Work out the finished part from the listing and answer in its coordinate system (mm). A direction names the side the tool comes from. Round coordinates to 2 decimals unless told otherwise and drop trailing zeros. Write each loop counter-clockwise with the first axis right and the second up, starting at its lowest first coordinate (ties: lowest second). Pieces come first, ordered by that corner, then holes.
1. A tool of negligible diameter and unlimited length cuts with its end or side. For faces 1 (the face through (-7, -27, 0)), 2 (the face through (3.724, 27.535, 3.697)), 3 (the face through (20, 0, 10)), 4 (the face through (21, -14, 15)), from which of +Z, -Z, +X, -X, +Y, -Y can it reach the whole face along a straight path? Write none if from no direction.
2. Find section A-A (y = -21). Write down the section's boundary in (x, z).
3. Straight lines are drawn through the part: probe 1 along Z at (x, y) = (-15, 28.15); probe 2 along Y at (x, z) = (-21, 17.75); probe 3 along Z at (x, y) = (-8, -26). For each, find the intervals that lie inside material, in ascending order.
4. Determine the mould class of faces 5 (the face through (-20.08, 27.54, 7.89)), 6 (the face through (-7, -27, 20)), 7 (the face through (43.5, -40, 12.6)) for opening direction X: pulls with the +X half, pulls with the -X half, needs draft (parallel to the pull), parting line crosses it, or undercut.
5. Flat-ended cylindrical pins translate along their axes: pin 1 Ø6 at (x, y) = (44, -2.5) entering from +Z; pin 2 Ø4 at (x, y) = (42, -36) entering from +Z; pin 3 Ø13 at (x, y) = (18.5, -38.5) entering from +Z. Find the tip coordinate at first contact, or state that the pin passes through.
6. Find section B-B (y = -83.5). Write down the section's boundary in (x, z), and give its area (3 significant figures).
```python
from build123d import *

# Parameters (mm, degrees)
BOSS_EXTRUDE2_DEPTH = 20
FILLET1_RADIUS      = 10
FILLET1_LENGTH      = 5
FILLET2_RADIUS      = 10
FILLET2_LENGTH      = 5
SKETCH5_R           = 1
SKETCH5_R_2         = 5.5
CUT_EXTRUDE5_DEPTH  = 69.007352544
CUT_EXTRUDE7_DEPTH  = 25
FILLET5_R           = 10
BOSS_EXTRUDE5_DEPTH = 60
SKETCH13_R          = 2.1
CUT_EXTRUDE8_DEPTH  = 60
BOSS_EXTRUDE6_START = 78
BOSS_EXTRUDE6_DEPTH = 78


with BuildPart() as part:
    # Sketch1 → Boss-Extrude2 (new body)
    with BuildSketch(Plane.XY):
        Polygon((-25, 30), (25, 30), (25, -30), (-25, -30), (-25, -25), (-20, -25), (20, -25), (20, 25), (-20, 25), (-25, 25), align=None)
    extrude(amount=BOSS_EXTRUDE2_DEPTH)

    # Fillet1: full round fillet: the end face becomes a half cylinder, R = half its width
    fillet1_face = Plane((-25, 27.5, 10), x_dir=(0, -1, 0), z_dir=(-1, 0, 0))  # on the end face: x along it, z out of the body
    fillet1_slab = fillet1_face.offset(-FILLET1_RADIUS / 2) * Box(FILLET1_LENGTH, 2 * FILLET1_RADIUS, FILLET1_RADIUS, mode=Mode.PRIVATE)  # the body's end, R deep
    fillet1_round = Plane((-15, 27.5, 10), x_dir=(-1, 0, 0), z_dir=(0, -1, 0)) * Cylinder(FILLET1_RADIUS, FILLET1_LENGTH, mode=Mode.PRIVATE)  # its axis R under the face
    add(fillet1_slab - fillet1_round, mode=Mode.SUBTRACT)

    # Fillet2: full round fillet: the end face becomes a half cylinder, R = half its width
    fillet2_face = Plane((-25, -27.5, 10), x_dir=(0, -1, 0), z_dir=(-1, 0, 0))  # on the end face: x along it, z out of the body
    fillet2_slab = fillet2_face.offset(-FILLET2_RADIUS / 2) * Box(FILLET2_LENGTH, 2 * FILLET2_RADIUS, FILLET2_RADIUS, mode=Mode.PRIVATE)  # the body's end, R deep
    fillet2_round = Plane((-15, -27.5, 10), x_dir=(-1, 0, 0), z_dir=(0, -1, 0)) * Cylinder(FILLET2_RADIUS, FILLET2_LENGTH, mode=Mode.PRIVATE)  # its axis R under the face
    add(fillet2_slab - fillet2_round, mode=Mode.SUBTRACT)

    # Sketch5 → Cut-Extrude5 (cut, through all)
    with BuildSketch(Plane(origin=(0, 30, 0), x_dir=(1, 0, 0), z_dir=(0, 1, 0))):
        with Locations(Location((-15, -3, 0), (0, 0, 180))):
            Circle(SKETCH5_R)
        with Locations(Location((-22, -10, 0), (0, 0, 180))):
            Circle(SKETCH5_R)
        with Locations(Location((-15, -17, 0), (0, 0, 180))):
            Circle(SKETCH5_R)
        with Locations(Location((-8, -10, 0), (0, 0, 180))):
            Circle(SKETCH5_R)
        with Locations(Location((-15, -10, 0), (0, 0, 180))):
            Circle(SKETCH5_R_2)
    extrude(amount=-CUT_EXTRUDE5_DEPTH, mode=Mode.SUBTRACT)

    # Sketch10 → Cut-Extrude7 (cut)
    with BuildSketch(Plane(origin=(25, 0, 0), x_dir=(0, 0, -1), z_dir=(1, 0, 0))):
        Polygon((-15, 28.180148829), (-15, -28.180148829), (-15, -30), (-20, -30), (-20, 30), (-15, 30), align=None)
        Polygon((-5, 28.180148829), (-5, -28.180148829), (-5, -30), (0, -30), (0, 30), (-5, 30), align=None)
    extrude(amount=-CUT_EXTRUDE7_DEPTH, mode=Mode.SUBTRACT)

    # Fillet5
    # the kernel refuses this fillet: 10 mm, written as the material it adds along each edge
    with BuildSketch(Plane(origin=(0, 25, 15), x_dir=(1, 0, 0), z_dir=(0, 1, 0)), Plane(origin=(0, -30, 15), x_dir=(1, 0, 0), z_dir=(0, 1, 0)), Plane(origin=(0, -25, 5), x_dir=(1, 0, 0), z_dir=(0, -1, 0))) as fillet5_piece_1:
        with BuildLine():
            CenterArc((8.660254038, -10), FILLET5_R, 90, 60)
            Line((0, -5), (-0.173205081, -4.9))
            ThreePointArc((-0.173205081, -4.9), (-0.2, -2.5), (-0.2, 0))
            Line((-0.2, 0), (0, 0.2))
            Line((0, 0.2), (8.660254038, 0.2))
            Line((8.660254038, 0.2), (8.660254038, 0))
        make_face()
    extrude(amount=5)
    with BuildSketch(Plane(origin=(0, 30, 5), x_dir=(0, 0, -1), z_dir=(0, -1, 0))) as fillet5_piece_2:
        with BuildLine():
            CenterArc((10, 8.660254038), FILLET5_R, 180, 60)
            Line((0, 8.660254038), (-0.2, 8.660254038))
            Line((-0.2, 8.660254038), (-0.2, 0))
            Line((-0.2, 0), (0, -0.2))
            ThreePointArc((0, -0.2), (2.5, -0.2), (4.9, -0.173205081))
            Line((4.9, -0.173205081), (5, 0))
        make_face()
    extrude(amount=5)

    # Sketch12 → Boss-Extrude5 (add)
    with BuildSketch(Plane.XZ.offset(30)):
        with BuildLine():
            Line((56.226298398, -3.359735054), (61.222506141, 5.302707337))
            ThreePointArc((61.222506141, 5.302707337), (43.74904955, 12.533728595), (25, 15))
            Line((25, 15), (25, 5))
            ThreePointArc((25, 5), (41.16297375, 2.873903962), (56.226298398, -3.359735054))
        make_face()
    extrude(amount=-BOSS_EXTRUDE5_DEPTH)

    # Sketch13 → Cut-Extrude8 (cut)
    with BuildSketch(Plane(origin=(2.920998947, 0, 10.910870277), x_dir=(-0.9659824633840055, 0, 0.2586075800021504), z_dir=(-0.2586075800021504, 0, -0.9659824633840055))):
        with Locations((-39.019497435, 15)):
            Circle(SKETCH13_R)
        with Locations((-39.019497435, 0)):
            Circle(SKETCH13_R)
        with Locations((-39.019497435, -15)):
            Circle(SKETCH13_R)
    extrude(amount=-CUT_EXTRUDE8_DEPTH, mode=Mode.SUBTRACT)

    # Sketch14 → Boss-Extrude6 (add)
    with BuildSketch(Plane.XZ.offset(30).offset(BOSS_EXTRUDE6_START)):
        with BuildLine():
            Line((61.222506141, 5.302707337), (56.226298398, -3.359735054))
            ThreePointArc((56.226298398, -3.359735054), (41.16297375, 2.873903962), (25, 5))
            Line((25, 5), (23.767457853, 5))
            Line((23.767457853, 5), (23.767457853, 15))
            Line((23.767457853, 15), (25, 15))
            ThreePointArc((25, 15), (43.74904955, 12.533728595), (61.222506141, 5.302707337))
        make_face()
    extrude(amount=-BOSS_EXTRUDE6_DEPTH)


solid = part.part
```
Worked answers:
1. face 1: -Z, -X, +Y, -Y
1. face 2: -Z, +Y, -Y
1. face 3: +Z, -Z, -X
1. face 4: +Z, +X, +Y, -Y
2. outline: (20, 5) - (25, 5) arc R62.5 cw to (56.23, -3.36) - (61.22, 5.3) arc R72.5 ccw to (25, 15) - (20, 15) - close
3. probe 1: z = 0 to 2, 4 to 4.5, 15.5 to 16, 18 to 20
3. probe 2: y = -30 to -25, 25 to 30
3. probe 3: z = 0 to 9, 11 to 20
4. face 5: undercut
4. face 6: needs draft
4. face 7: pulls with the +X half
5. pin 1: stops at z = 13.21
5. pin 2: stops at z = 13.43
5. pin 3: stops at z = 15
6. outline: (23.77, 5) - (25, 5) arc R62.5 cw to (56.23, -3.36) - (61.22, 5.3) arc R72.5 ccw to (25, 15) - (23.77, 15) - close
6. area: 365 mm2
